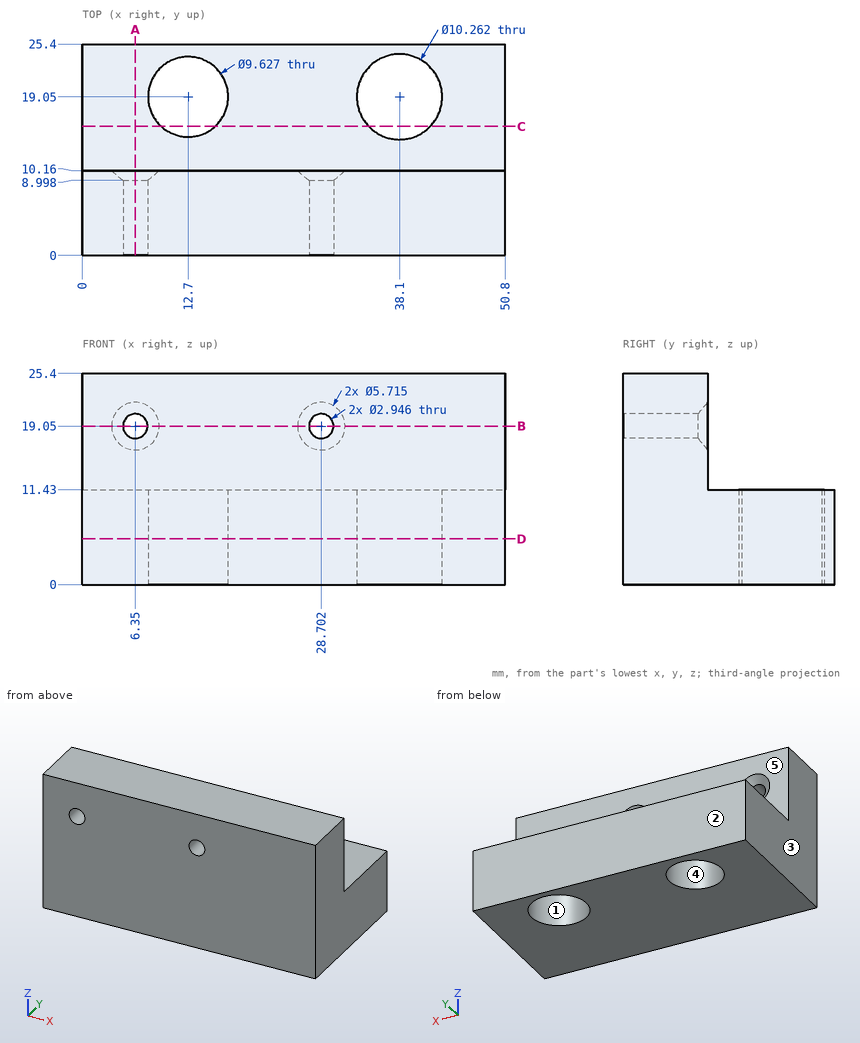
Verification items for this drawing (mm, ordinates from the low corner). A direction names the side the tool comes from. Coordinates: 2 decimals unless noted, no trailing zeros. Write each loop counter-clockwise with the first axis right and the second up, starting at its lowest first coordinate (ties: lowest second). Pieces come first, ordered by that corner, then holes. Notation, with made-up numbers: M 58.25,13.5 L 89.25,13.5 A22 cw 89.25,46.5 Z; hole C 14,0.5 d5. An arc over 180 degrees is marked long. Answer as a JSON object with one key per item and string values. Group by question number.
(1) Cross-section at B-B, the plane z = 19.05. Record the cut outline in (x, y) (1 decimal), and give its area (3 significant figures).
(2) Gauge pin test, flat ends, axial feed: pin 1 (5 mm diameter, centred on x = 45.5, z = 20.5, fed in from +Y); pin 2 (1.8 mm diameter, centred on x = 6.35, z = 19.05, fed in from +Y). Record the tip position at first contact, or that the pin passes through.
(3) Tool access check on the marked faces 4 and 5. Record the directions out of +Z, -Z, +X, -X, +Y, -Y that give a thin tool (end or side, any length) a straight path to the whole face; none if there is none.
(4) Cross-section at A-A, the plane x = 6.35. Record the cut outline in (y, z), and give its area (3 significant figures).
(5) Cross-section at D-D, the plane z = 5.5. Record the cut outline in (x, y), and give its area (4 significant figures).
(6) Material ranges on line 1 (X direction, y = 3, z = 19.05) (1 decimal); line 2 (Y direction, x = 12.7, z = 7.5); line 3 (Y direction, x = 15.5, z = 20.25), recorded low to high.
(7) Release check for a two-part mould opening along X. For the marked faces 1, 2 and 3 record: +X half, -X half, draft (parallel to the pull), parting line (faces both ways), or undercut.
(8) Cross-section at C-C, the plane y = 15.5. State how many separate pieces and enclosed holes the cut face has, and give its area (3 significant figures).
Reply:
{
 "1": {"outline": "M 0,0 L 4.9,0 L 4.9,9 L 3.5,10.2 L 0,10.2 Z; M 7.8,0 L 27.2,0 L 27.2,9 L 25.8,10.2 L 9.2,10.2 L 7.8,9 Z; M 30.2,0 L 50.8,0 L 50.8,10.2 L 31.6,10.2 L 30.2,9 Z", "area": "453 mm²"},
 "2": {"pin 1": "y = 10.16", "pin 2": "through"},
 "3": {"face 4": "+Z, -Z", "face 5": "+Z, +X, -X, +Y"},
 "4": {"outline": "M 0,0 L 25.4,0 L 25.4,11.43 L 10.16,11.43 L 10.16,16.19 L 9,17.58 L 0,17.58 Z; M 0,20.52 L 9,20.52 L 10.16,21.91 L 10.16,25.4 L 0,25.4 Z", "area": "401 mm²"},
 "5": {"outline": "M 0,0 L 50.8,0 L 50.8,25.4 L 0,25.4 Z; hole C 12.7,19.05 d9.63; hole C 38.1,19.05 d10.26", "area": "1,135 mm²"},
 "6": {"line 1": "0 to 4.9, 7.8 to 27.2, 30.2 to 50.8", "line 2": "0 to 14.24, 23.86 to 25.4", "line 3": "0 to 10.16"},
 "7": {"face 1": "undercut", "face 2": "draft", "face 3": "-X half"},
 "8": {"separate pieces": "3", "enclosed holes": "0", "area": "422 mm²"}
}
